from build123d import *

# Parameters (mm, degrees)
F0_R       = 10
F1_DEPTH   = 10
F1_FACE1_R = 10
F2_R       = 7
F4_DEPTH   = 10
F5_T       = -2
F6_R       = 5
F7_DEPTH   = 2


with BuildPart() as f1:
    # F0 (on Front) → F1 (new body)
    with BuildSketch(Plane.XZ):
        Circle(F0_R)
    extrude(amount=F1_DEPTH)

    # F1_face1 (on face) → F3 section 0
    with BuildSketch(Plane.XZ.offset(10)):
        Circle(F1_FACE1_R)
    # F2 (on face) → F3 section 1
    with BuildSketch(Plane(origin=(0, 0, 0), x_dir=(-1, 0, 0), z_dir=(0, 1, 0))):
        Circle(F2_R)
    loft(mode=Mode.INTERSECT)

    # F4 (add): a face of the model
    f4_faces = [f1.faces().sort_by_distance(p)[0] for p in [
        (0, -10, 0),
    ]]
    extrude(f4_faces, amount=F4_DEPTH)

    # F5
    f5_openings = [f1.faces().sort_by_distance(p)[0] for p in [
        (0, -20, 0),
    ]]
    offset(amount=F5_T, openings=f5_openings)

    # F6 (on face) → F7 (cut)
    with BuildSketch(Plane(origin=(0, 0, 0), x_dir=(-1, 0, 0), z_dir=(0, 1, 0))):
        Circle(F6_R)
    extrude(amount=-F7_DEPTH, mode=Mode.SUBTRACT)


solid = f1.part
Geometry: final body of the model. Coordinates: model frame, mm. A direction names the side the tool comes from. Coordinates: 2 decimals unless noted, no trailing zeros. Order: outer loops, then holes, each group sorted by start corner. A loop starts at its lowest first (then second) coordinate and runs counter-clockwise, first axis right, second up.
(1) Material intervals for probe 1 along X at (y, z) = (-14, 0); probe 2 along Z at (x, y) = (3.75, -14.5), sorted ascending.
(2) Draft query along X for faces 1 (the face through (9.54, -14.93, -3)), 2 (the face through (-4.909, -4.246, -3.764)), 3 (the face through (0, -20, 8.2)). Return one class per face: pulls with the +X half, pulls with the -X half, needs draft (parallel to the pull), parting line crosses it, or undercut.
(3) Access query for faces 4 (the face through (1.08, -0.99, -4.88)), 5 (the face through (-1.6, -2, -4.9)). Directions: +Z, -Z, +X, -X, +Y, -Y. A direction counts if a zero-diameter tool reaches every point of the face in a straight line with its end or side. Return the directions, or none.
(4) Section query B-B (y = -17). Return the cut outline in (x, z).
(5) Section query A-A (x = 0). Return the cut outline in (y, z), plus the area to 3 significant figures.
(6) Section query C-C (y = -9). Return the cut outline in (x, z), plus the area to 3 significant figures.
(7) First-contact query: pin 1 (1 mm diameter, centred on y = -9, z = 2, fed in from -X); pin 2 (4 mm diameter, centred on y = -6.5, z = -5.5, fed in from +X); pin 3 (6 mm diameter, centred on x = 0, z = 0, fed in from -Y); pin 4 (2 mm diameter, centred on x = -6, y = -16.5, fed in from -Z). Flat tips, straight axial feed; report the tip coordinate or a pass-through.
Solution:
1. probe 1: x = -10 to -8, 8 to 10
1. probe 2: z = -9.27 to -7.07, 7.07 to 9.27
2. face 1: parting line crosses it
2. face 2: undercut
2. face 3: needs draft
3. face 4: +Y, -Y
3. face 5: -Y
4. outline: circle Ø20 at (0, 0); hole circle Ø16 at (0, 0)
5. outline: (-20, -10) - (-10, -10) - (0, -7) - (0, -5) - (-2, -5) - (-2, -5.51) - (-10.29, -8) - (-20, -8) - close; (-20, 8) - (-10.29, 8) - (-2, 5.51) - (-2, 5) - (0, 5) - (0, 7) - (-10, 10) - (-20, 10) - close
5. area: 82.6 mm2
6. outline: circle Ø19.4 at (0, 0); hole circle Ø15.22 at (0, 0)
6. area: 114 mm2
7. pin 1: stops at x = -9.67
7. pin 2: stops at x = 8.45
7. pin 3: passes through
7. pin 4: stops at z = -8.66
